Input: part model. Units: mm. Frame: model coordinates. A direction names the side the tool comes from. Coordinates: 2 decimals unless noted, no trailing zeros. Loops run counter-clockwise (first coordinate to the right, second up) from the corner with the lowest first, then second, coordinate; pieces in that order, holes last.
```python
from build123d import *

# Parameters (mm, degrees)
SKETCH1_W             = 50
SKETCH1_H             = 25
BOSS_EXTRUDE1_DEPTH   = 4
SKETCH2_W             = 50
SKETCH2_H             = 22
BOSS_EXTRUDE2_DEPTH   = 4
SKETCH3_R             = 8.0645
CUT_EXTRUDE1_DEPTH    = 23
SKETCH4_R             = 2
BOSS_EXTRUDE4_DEPTH   = 5
F_3_0MM_DOWEL_HOLE1_D = 3
F_2_0MM_DOWEL_HOLE1_D = 2
MIRROR4_COPY_1_D      = 2
FILLET1_R             = 10
FILLET2_R             = 5


with BuildPart() as part:
    # Sketch1 → Boss-Extrude1 (new body)
    with BuildSketch(Plane.XY):
        Rectangle(SKETCH1_W, SKETCH1_H)
    extrude(amount=BOSS_EXTRUDE1_DEPTH)

    # Sketch2 → Boss-Extrude2 (add)
    with BuildSketch(Plane.XZ.offset(12.5)):
        with Locations((0, -7)):
            Rectangle(SKETCH2_W, SKETCH2_H)
    extrude(amount=BOSS_EXTRUDE2_DEPTH)

    # Sketch3 → Cut-Extrude1 (cut, through all)
    with BuildSketch(Plane.XY.offset(4)):
        with Locations((13.2715, 0)):
            Circle(SKETCH3_R)
    cut_extrude1 = extrude(amount=-CUT_EXTRUDE1_DEPTH, mode=Mode.SUBTRACT)

    # Mirror1: Cut-Extrude1 across plane
    add(cut_extrude1.mirror(Plane(origin=(0, 0, 0), x_dir=(0, 0, 1), z_dir=(1, 0, 0))), mode=Mode.SUBTRACT)

    # Sketch4 → Boss-Extrude4 (add)
    with BuildSketch(Plane(origin=(0, 0, 0), x_dir=(-1, 0, 0), z_dir=(0, 0, -1))):
        Circle(SKETCH4_R)
    extrude(amount=BOSS_EXTRUDE4_DEPTH)

    # Ø3.0mm Dowel Hole1 (through all)
    with Locations(Plane(origin=(0, -12.5, 0), x_dir=(1, 0, 0), z_dir=(0, 1, 0))):
        with Locations((-20, 13)):
            f_3_0mm_dowel_hole1 = Hole(F_3_0MM_DOWEL_HOLE1_D / 2)

    # Mirror2: Ø3.0mm Dowel Hole1 across plane
    add(f_3_0mm_dowel_hole1.mirror(Plane(origin=(0, 0, 0), x_dir=(0, 0, 1), z_dir=(1, 0, 0))), mode=Mode.SUBTRACT)

    # Ø2.0mm Dowel Hole1 (through all)
    with Locations(Plane(origin=(0, 0, 0), x_dir=(-1, 0, 0), z_dir=(0, 0, -1))):
        with Locations((-21, 8.5)):
            f_2_0mm_dowel_hole1 = Hole(F_2_0MM_DOWEL_HOLE1_D / 2)

    # Mirror3: Ø2.0mm Dowel Hole1 across plane
    add(f_2_0mm_dowel_hole1.mirror(Plane.ZX), mode=Mode.SUBTRACT)

    # Mirror4: Ø2.0mm Dowel Hole1 across plane
    add(f_2_0mm_dowel_hole1.mirror(Plane(origin=(0, 0, 0), x_dir=(0, 0, 1), z_dir=(1, 0, 0))), mode=Mode.SUBTRACT)

    # Mirror4 copy 1 (through all)
    with Locations(Plane(origin=(0, 0, 0), x_dir=(1, 0, 0), z_dir=(0, 0, -1))):
        with Locations((-21, 8.5)):
            Hole(MIRROR4_COPY_1_D / 2)

    # Fillet1
    fillet1_edges = [part.edges().sort_by_distance(p)[0] for p in [
        (-25, -14.5, -18),
        (25, -14.5, -18),
    ]]
    fillet(fillet1_edges, radius=FILLET1_R)

    # Fillet2
    fillet2_edges = [part.edges().sort_by_distance(p)[0] for p in [
        (-25, 12.5, 2),
        (25, 12.5, 2),
    ]]
    fillet(fillet2_edges, radius=FILLET2_R)


solid = part.part
```
Item 1: Section query A-A (z = 2.5). Output: boundary loops of the cut face in (x, y), then the cut area to 3 significant figures.
Result:
outline: (-25, -16.5) - (25, -16.5) - (25, 7.5) arc R5 ccw to (20, 12.5) - (-20, 12.5) arc R5 ccw to (-25, 7.5) - close; hole circle Ø2 at (-21, -8.5); hole circle Ø2 at (-21, 8.5); hole circle Ø16.13 at (-13.27, 0); hole circle Ø16.13 at (13.27, 0); hole circle Ø2 at (21, -8.5); hole circle Ø2 at (21, 8.5)
area: 1,020 mm2
Item 2: Section query B-B (y = 0). Output: boundary loops of the cut face in (x, z).
Result:
outline: (-25, 0) - (-21.34, 0) - (-21.34, 4) - (-25, 4) - close; (-5.21, 0) - (-2, 0) - (-2, -5) - (2, -5) - (2, 0) - (5.21, 0) - (5.21, 4) - (-5.21, 4) - close; (21.34, 0) - (25, 0) - (25, 4) - (21.34, 4) - close
Item 3: Section query D-D (x = -10.5). Output: boundary loops of the cut face in (y, z), then the cut area to 3 significant figures.
Result:
outline: (-16.5, -18) - (-12.5, -18) - (-12.5, 0) - (-7.57, 0) - (-7.57, 4) - (-16.5, 4) - close; (7.57, 0) - (12.5, 0) - (12.5, 4) - (7.57, 4) - close
area: 127 mm2
Item 4: Section query C-C (z = -1.5). Output: boundary loops of the cut face in (x, y), then the cut area to 3 significant figures.
Result:
outline: (-25, -16.5) - (25, -16.5) - (25, -12.5) - (-25, -12.5) - close; circle Ø4 at (0, 0)
area: 213 mm2
Item 5: Reachability of faces 1 (the face through (0, 0, -5)), 2 (the face through (0, -2, -2)), 3 (the face through (0, -16.5, -7)) from +Z, -Z, +X, -X, +Y, -Y: full face, straight path, thin tool, end or side. Return the list, or none.
Result:
face 1: -Z, +X, -X, +Y
face 2: -Z
face 3: +Z, -Z, +X, -X, -Y
Item 6: Line query: L1, parallel to X at y = 0.5, z = 1.5; L2, parallel to X at y = 2, z = 0.25; L3, parallel to Y at x = 13, z = 2. Output: solid intervals per line, ascending.
Result:
L1: x = -25 to -21.32, -5.22 to 5.22, 21.32 to 25
L2: x = -25 to -21.08, -5.46 to 5.46, 21.08 to 25
L3: y = -16.5 to -8.06, 8.06 to 12.5
Item 7: Contact query for flat-ended pins moving along their axis: P1, Ø1.2, axis at x = 21, y = 8.5, coming from the +Z side; P2, Ø3, axis at x = 21, y = -8.5, coming from the -Z side; P3, Ø4.5, axis at x = 0, y = -0.5, coming from the -Z side; P4, Ø1, axis at x = -4.5, z = -2.5, coming from the +Y side. Output: stop coordinate, or through.
Result:
P1: passes through
P2: stops at z = 0
P3: stops at z = -5
P4: stops at y = -12.5
Item 8: Mould query, pull axis Y, two halves, no side actions, for faces 4 (the face through (23.5, 11.07, 2.03)), 5 (the face through (-5.215, 0.355, 2.028)), 6 (the face through (-25, -7, 1)). Classes: +Y half, -Y half, draft (parallel to the pull), parting line (faces both ways), or undercut.
Result:
face 4: +Y half
face 5: undercut
face 6: draft
